Part model, mm, in its own coordinate system. Face numbers are marked on the shaded views. A direction names the side the tool comes from. Give positions to 0.01 mm unless a question says otherwise; leave off trailing zeros. Loops run counter-clockwise (first coordinate to the right, second up) from the corner with the lowest first, then second, coordinate; pieces in that order, holes last. Notation, with made-up numbers: (11.25, 53.5) -> (54.25, 53.5) arc R35 cw to (54.25, 86.5) -> close; hole circle Ø4 at (75.5, 10.5). An arc over 180 degrees is marked (long way). Write item = value, one per line.
from build123d import *

# Parameters (mm, degrees)
F1_DEPTH = 2
F2_R     = 1
F3_DEPTH = 2.001


with BuildPart() as f1:
    # F0 (on Top) → F1 (new body)
    with BuildSketch(Plane.XY):
        with BuildLine():
            ThreePointArc((12.498086, -0.218737), (12.499521, -0.109373), (12.5, 0))
            ThreePointArc((12.5, 0), (12.419615, 1.415329), (12.179495, 2.812455))
            ThreePointArc((12.179495, 2.812455), (11.888206, 3.862712), (11.506538, 4.883604))
            ThreePointArc((11.506538, 4.883604), (10.825318, 6.25), (9.982594, 7.523152))
            ThreePointArc((9.982594, 7.523152), (9.28931, 8.364133), (8.525405, 9.141525))
            ThreePointArc((8.525405, 9.141525), (7.347316, 10.112712), (6.059612, 10.933028))
            ThreePointArc((6.059612, 10.933028), (5.084208, 11.419318), (4.070152, 11.818793))
            ThreePointArc((4.070152, 11.818793), (2.598896, 12.226845), (1.088867, 12.452484))
            ThreePointArc((1.088867, 12.452484), (0, 12.5), (-1.088867, 12.452484))
            ThreePointArc((-1.088867, 12.452484), (-2.598896, 12.226845), (-4.070152, 11.818793))
            ThreePointArc((-4.070152, 11.818793), (-5.084208, 11.419318), (-6.059612, 10.933028))
            ThreePointArc((-6.059612, 10.933028), (-7.347316, 10.112712), (-8.525405, 9.141525))
            ThreePointArc((-8.525405, 9.141525), (-9.28931, 8.364133), (-9.982594, 7.523152))
            ThreePointArc((-9.982594, 7.523152), (-10.825318, 6.25), (-11.506538, 4.883604))
            ThreePointArc((-11.506538, 4.883604), (-11.888206, 3.862712), (-12.179495, 2.812455))
            ThreePointArc((-12.179495, 2.812455), (-12.431524, 1.306606), (-12.498086, -0.218737))
            ThreePointArc((-12.498086, -0.218737), (-12.431524, -1.306606), (-12.270451, -2.384541))
            ThreePointArc((-12.270451, -2.384541), (-11.888206, -3.862712), (-11.328602, -5.283255))
            ThreePointArc((-11.328602, -5.283255), (-10.825318, -6.25), (-10.239734, -7.169229))
            ThreePointArc((-10.239734, -7.169229), (-9.28931, -8.364133), (-8.200299, -9.434251))
            ThreePointArc((-8.200299, -9.434251), (-7.347316, -10.112712), (-6.438475, -10.714292))
            ThreePointArc((-6.438475, -10.714292), (-5.084208, -11.419318), (-3.65409, -11.953979))
            ThreePointArc((-3.65409, -11.953979), (-2.598896, -12.226845), (-1.523944, -12.406756))
            ThreePointArc((-1.523944, -12.406756), (0, -12.5), (1.523944, -12.406756))
            ThreePointArc((1.523944, -12.406756), (2.598896, -12.226845), (3.65409, -11.953979))
            ThreePointArc((3.65409, -11.953979), (5.084208, -11.419318), (6.438475, -10.714292))
            ThreePointArc((6.438475, -10.714292), (7.347316, -10.112712), (8.200299, -9.434251))
            ThreePointArc((8.200299, -9.434251), (9.28931, -8.364133), (10.239734, -7.169229))
            ThreePointArc((10.239734, -7.169229), (10.825318, -6.25), (11.328602, -5.283255))
            ThreePointArc((11.328602, -5.283255), (11.888206, -3.862712), (12.270451, -2.384541))
            ThreePointArc((12.270451, -2.384541), (12.431524, -1.306606), (12.498086, -0.218737))
        make_face()
        with BuildLine():
            ThreePointArc((11.506538, 4.883604), (11.888206, 3.862712), (12.179495, 2.812455))
            ThreePointArc((12.179495, 2.812455), (13.150138, 3.278627), (13.944828, 4.005218))
            Line((13.944828, 4.005218), (13.790319, 4.480746))
            Line((13.790319, 4.480746), (13.635811, 4.956275))
            ThreePointArc((13.635811, 4.956275), (12.565814, 5.076992), (11.506538, 4.883604))
        make_face()
        with BuildLine():
            ThreePointArc((14.472832, -1.018402), (13.544441, -0.472914), (12.498086, -0.218737))
            ThreePointArc((12.498086, -0.218737), (12.431524, -1.306606), (12.270451, -2.384541))
            ThreePointArc((12.270451, -2.384541), (13.346787, -2.353468), (14.368303, -2.012924))
            Line((14.368303, -2.012924), (14.420567, -1.515663))
            Line((14.420567, -1.515663), (14.472832, -1.018402))
        make_face()
        with BuildLine():
            ThreePointArc((8.525405, 9.141525), (9.28931, 8.364133), (9.982594, 7.523152))
            ThreePointArc((9.982594, 7.523152), (10.679711, 8.343818), (11.110165, 9.330821))
            Line((11.110165, 9.330821), (10.7756, 9.702394))
            Line((10.7756, 9.702394), (10.441035, 10.073966))
            ThreePointArc((10.441035, 10.073966), (9.414444, 9.74904), (8.525405, 9.141525))
        make_face()
        with BuildLine():
            ThreePointArc((12.807368, -6.816987), (12.181111, -5.941049), (11.328602, -5.283255))
            ThreePointArc((11.328602, -5.283255), (10.825318, -6.25), (10.239734, -7.169229))
            ThreePointArc((10.239734, -7.169229), (11.235655, -7.578627), (12.307368, -7.683013))
            Line((12.307368, -7.683013), (12.557368, -7.25))
            Line((12.557368, -7.25), (12.807368, -6.816987))
        make_face()
        with BuildLine():
            ThreePointArc((4.070152, 11.818793), (5.084208, 11.419318), (6.059612, 10.933028))
            ThreePointArc((6.059612, 10.933028), (6.362665, 11.966287), (6.354454, 13.043041))
            Line((6.354454, 13.043041), (5.897681, 13.246409))
            Line((5.897681, 13.246409), (5.440909, 13.449777))
            ThreePointArc((5.440909, 13.449777), (4.635231, 12.735391), (4.070152, 11.818793))
        make_face()
        with BuildLine():
            ThreePointArc((8.927395, -11.436854), (8.711557, -10.381923), (8.200299, -9.434251))
            ThreePointArc((8.200299, -9.434251), (7.347316, -10.112712), (6.438475, -10.714292))
            ThreePointArc((6.438475, -10.714292), (7.181776, -11.493373), (8.118378, -12.024639))
            Line((8.118378, -12.024639), (8.522886, -11.730746))
            Line((8.522886, -11.730746), (8.927395, -11.436854))
        make_face()
        with BuildLine():
            ThreePointArc((-1.088867, 12.452484), (0, 12.5), (1.088867, 12.452484))
            ThreePointArc((1.088867, 12.452484), (0.945456, 13.519676), (0.5, 14.5))
            Line((0.5, 14.5), (0, 14.5))
            Line((0, 14.5), (-0.5, 14.5))
            ThreePointArc((-0.5, 14.5), (-0.945456, 13.519676), (-1.088867, 12.452484))
        make_face()
        with BuildLine():
            ThreePointArc((3.503793, -14.079184), (3.735695, -13.027668), (3.65409, -11.953979))
            ThreePointArc((3.65409, -11.953979), (2.598896, -12.226845), (1.523944, -12.406756))
            ThreePointArc((1.523944, -12.406756), (1.886103, -13.42081), (2.525646, -14.287096))
            Line((2.525646, -14.287096), (3.01472, -14.18314))
            Line((3.01472, -14.18314), (3.503793, -14.079184))
        make_face()
        with BuildLine():
            ThreePointArc((-6.059612, 10.933028), (-5.084208, 11.419318), (-4.070152, 11.818793))
            ThreePointArc((-4.070152, 11.818793), (-4.635231, 12.735391), (-5.440909, 13.449777))
            Line((-5.440909, 13.449777), (-5.897681, 13.246409))
            Line((-5.897681, 13.246409), (-6.354454, 13.043041))
            ThreePointArc((-6.354454, 13.043041), (-6.362665, 11.966287), (-6.059612, 10.933028))
        make_face()
        with BuildLine():
            ThreePointArc((-2.525646, -14.287096), (-1.886103, -13.42081), (-1.523944, -12.406756))
            ThreePointArc((-1.523944, -12.406756), (-2.598896, -12.226845), (-3.65409, -11.953979))
            ThreePointArc((-3.65409, -11.953979), (-3.735695, -13.027668), (-3.503793, -14.079184))
            Line((-3.503793, -14.079184), (-3.01472, -14.18314))
            Line((-3.01472, -14.18314), (-2.525646, -14.287096))
        make_face()
        with BuildLine():
            ThreePointArc((-9.982594, 7.523152), (-9.28931, 8.364133), (-8.525405, 9.141525))
            ThreePointArc((-8.525405, 9.141525), (-9.414444, 9.74904), (-10.441035, 10.073966))
            Line((-10.441035, 10.073966), (-10.7756, 9.702394))
            Line((-10.7756, 9.702394), (-11.110165, 9.330821))
            ThreePointArc((-11.110165, 9.330821), (-10.679711, 8.343818), (-9.982594, 7.523152))
        make_face()
        with BuildLine():
            ThreePointArc((-8.118378, -12.024639), (-7.181776, -11.493373), (-6.438475, -10.714292))
            ThreePointArc((-6.438475, -10.714292), (-7.347316, -10.112712), (-8.200299, -9.434251))
            ThreePointArc((-8.200299, -9.434251), (-8.711557, -10.381923), (-8.927395, -11.436854))
            Line((-8.927395, -11.436854), (-8.522886, -11.730746))
            Line((-8.522886, -11.730746), (-8.118378, -12.024639))
        make_face()
        with BuildLine():
            ThreePointArc((-12.179495, 2.812455), (-11.888206, 3.862712), (-11.506538, 4.883604))
            ThreePointArc((-11.506538, 4.883604), (-12.565814, 5.076992), (-13.635811, 4.956275))
            Line((-13.635811, 4.956275), (-13.790319, 4.480746))
            Line((-13.790319, 4.480746), (-13.944828, 4.005218))
            ThreePointArc((-13.944828, 4.005218), (-13.150138, 3.278627), (-12.179495, 2.812455))
        make_face()
        with BuildLine():
            ThreePointArc((-12.307368, -7.683013), (-11.235655, -7.578627), (-10.239734, -7.169229))
            ThreePointArc((-10.239734, -7.169229), (-10.825318, -6.25), (-11.328602, -5.283255))
            ThreePointArc((-11.328602, -5.283255), (-12.181111, -5.941049), (-12.807368, -6.816987))
            Line((-12.807368, -6.816987), (-12.557368, -7.25))
            Line((-12.557368, -7.25), (-12.307368, -7.683013))
        make_face()
        with BuildLine():
            ThreePointArc((-12.270451, -2.384541), (-12.431524, -1.306606), (-12.498086, -0.218737))
            ThreePointArc((-12.498086, -0.218737), (-13.544441, -0.472914), (-14.472832, -1.018402))
            Line((-14.472832, -1.018402), (-14.420567, -1.515663))
            Line((-14.420567, -1.515663), (-14.368303, -2.012924))
            ThreePointArc((-14.368303, -2.012924), (-13.346787, -2.353468), (-12.270451, -2.384541))
        make_face()
    extrude(amount=F1_DEPTH)

    # F2 (on face) → F3 (cut, through all)
    with BuildSketch(Plane.XY.offset(2)):
        Circle(F2_R)
    extrude(amount=-F3_DEPTH, mode=Mode.SUBTRACT)


solid = f1.part
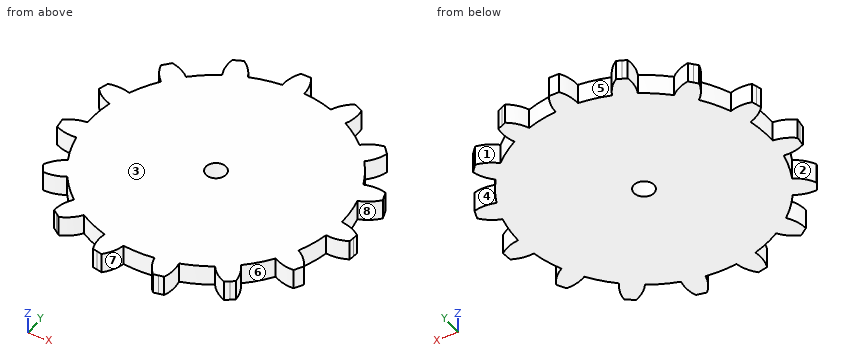
1) Pull direction X, two halves, no side cores. Call the marked faces 1, 2, 3 and 4: pulls with the +X half, pulls with the -X half, needs draft (parallel to the pull), parting line crosses it, or undercut.
Resolved:
face_1 = undercut
face_2 = pulls with the -X half
face_3 = needs draft
face_4 = undercut
2) Slice it at B-B, the plane y = -2.75. List the corners of the cut face in (x, z), and give its area (3 significant figures).
Resolved:
outline = (-12.19, 0) -> (12.19, 0) -> (12.19, 2) -> (-12.19, 2) -> close
area = 48.8 mm²
3) Drill centre lines: line 1 along Y through (x, z) = (0, 0.8); line 2 along X through (y, z) = (9.75, 0.8); line 3 along X through (y, z) = (12.5, 0.7). Where is each one in solid material? Low to high. Write a range as [from, to].
Resolved:
line_1 = [-12.5, -1], [1, 14.5]
line_2 = [-10.73, -9.42], [-7.82, 7.82], [9.42, 10.73]
line_3 = [-6.4, -4.45], [-1.09, 1.09], [4.45, 6.4]
4) Which spindle directions (+Z, -Z, +X, -X, +Y, -Y) get a long thin tool onto all of the face, cutting with end or side? Do the marked faces 5, 6, 7 and 8. Say none if no direction does.
Resolved:
face_5 = +Z, -Z, +Y
face_6 = +Z, -Z
face_7 = +Z, -Z, -Y
face_8 = +Z, -Z, +X
5) Drop flat-ended pins along their axis: P1, Ø1, axis at x = -7, y = 8.5, coming from the -Z side; P2, Ø1, axis at y = 10, z = 1, coming from the -X side. Give the stop position or say it passes through.
Resolved:
P1 = 0
P2 = -10.96
6) Slice it at A-A, the plane x = 0. List the corners of the cut face in (y, z).
Resolved:
outline = (-12.5, 0) -> (-1, 0) -> (-1, 2) -> (-12.5, 2) -> close; (1, 0) -> (14.5, 0) -> (14.5, 2) -> (1, 2) -> close
